Autodesk Inventor part; units mm, degrees
ref_plane "YZ Plane" through (0, 0, 0) normal (1, 0, 0) x (0, 1, 0)
ref_plane "XZ Plane" through (0, 0, 0) normal (0, 1, 0) x (-1, 0, 0)
ref_plane "XY Plane" through (0, 0, 0) normal (0, 0, 1) x (1, 0, 0)
sketch "Esquisse1" plane through (0, 0, 0) normal (0, 0, 1) x (1, 0, 0)
  line L0 (0, 0) -> (100, 0)
  line L1 (100, 0) -> (100, 80)
  line L2 (100, 80) -> (0, 80)
  line L3 (0, 80) -> (0, 0)
  dimension "d0" = 100
  dimension "d1" = 80
extrude "Extrusion1" add sketch "Esquisse1" against normal blind 5
sketch "Esquisse7" plane through (0, 0, 0) normal (0, 0, 1) x (1, 0, 0)
  line L0 (0, 0) -> (0, 45)
  line L1 (0, 0) -> (0, 80)
  line L2 (0, 45) -> (100, 45)
  line L3 (50, 45) -> (10, 45)
  line L4 (50, 45) -> (90, 45)
  line L5 (10, 45) -> (13, 45)
  line L6 (13, 45) -> (13, 50)
  line L7 (13, 50) -> (10, 50)
  line L8 (10, 50) -> (10, 45)
  line L9 (90, 45) -> (87, 45)
  line L10 (87, 45) -> (87, 50)
  line L11 (87, 50) -> (90, 50)
  line L12 (90, 50) -> (90, 45)
  line L13 (50, 45) -> (52.5, 45)
  line L14 (52.5, 45) -> (52.5, 50)
  line L15 (52.5, 50) -> (47.5, 50)
  line L16 (47.5, 50) -> (47.5, 45)
  line L17 (50, 45) -> (47.5, 45)
  line L18 (86.75, 44.75) -> (90.25, 44.75)
  line L19 (90.25, 44.75) -> (90.25, 50.25)
  line L20 (90.25, 50.25) -> (86.75, 50.25)
  line L21 (86.75, 50.25) -> (86.75, 44.75)
  line L22 (86.75, 44.75) -> (90.25, 50.25) construction
  line L23 (90.25, 44.75) -> (86.75, 50.25) construction
  line L24 (47.25, 44.75) -> (52.75, 44.75)
  line L25 (52.75, 44.75) -> (52.75, 50.25)
  line L26 (52.75, 50.25) -> (47.25, 50.25)
  line L27 (47.25, 50.25) -> (47.25, 44.75)
  line L28 (47.25, 44.75) -> (52.75, 50.25) construction
  line L29 (52.75, 44.75) -> (47.25, 50.25) construction
  line L30 (9.75, 44.75) -> (13.25, 44.75)
  line L31 (13.25, 44.75) -> (13.25, 50.25)
  line L32 (13.25, 50.25) -> (9.75, 50.25)
  line L33 (9.75, 50.25) -> (9.75, 44.75)
  line L34 (9.75, 44.75) -> (13.25, 50.25) construction
  line L35 (13.25, 44.75) -> (9.75, 50.25) construction
  point P0 (87, 45)
  point P1 (13, 45)
  point P2 (52.5, 45)
  point P3 (88.5, 47.5)
  point P4 (50, 47.5)
  point P5 (11.5, 47.5)
  point P6 (90.25, 45)
  point P7 (86.75, 45)
  point P8 (52.75, 45)
  point P9 (47.25, 45)
  point P10 (13.25, 45)
  point P11 (9.75, 45)
  point P12 (87, 45.05)
  point P13 (90, 45.05)
  dimension "d42" = 45
  dimension "d43" = 100
  dimension "d44" = 40
  dimension "d45" = 40
  dimension "d46" = 3
  dimension "d47" = 5
  dimension "d48" = 3
  dimension "d49" = 5
  dimension "d53" = 2.5
  dimension "d54" = 5
  dimension "d55" = 5
  dimension "d56" = 3.5
  dimension "d57" = 5.5
  dimension "d58" = 5.5
  dimension "d59" = 3.5
  dimension "d60" = 5.5
  dimension "d61" = 5.5
extrude "Extrusion2" cut sketch "Esquisse7" against normal through all
sketch "Esquisse8" plane through (0, 0, 0) normal (0, 0, 1) x (1, 0, 0)
  line L0 (0, 0) -> (0, 40)
  line L1 (0, 0) -> (0, 80)
  line L2 (0, 40) -> (50, 40)
  line L3 (100, 80) -> (100, 0)
  line L4 (-5, -5) -> (105, -5)
  line L5 (105, -5) -> (105, 85)
  line L6 (105, 85) -> (-5, 85)
  line L7 (-5, 85) -> (-5, -5)
  line L8 (-5, -5) -> (105, 85) construction
  line L9 (105, -5) -> (-5, 85) construction
  line L10 (100, 80) -> (0, 80)
  line L11 (0, 80) -> (0, 0)
  line L12 (0, 0) -> (100, 0)
  line L13 (100, 0) -> (100, 80)
  dimension "d62" = 40
  dimension "d63" = 50
  dimension "d64" = 110
  dimension "d65" = 90
extrude "Extrusion3" add sketch "Esquisse8" against normal blind 5
sketch "Esquisse9" plane through (0, 0, 0) normal (0, 0, 1) x (1, 0, 0)
  line L0 (0, 0) -> (-0.05, 0)
  line L1 (-0.05, 0) -> (-0.05, -0.95)
  line L2 (-0.05, -0.95) -> (20.05, -0.95)
  line L3 (20.05, -0.95) -> (20.05, -4.05)
  line L4 (20.05, -4.05) -> (-0.05, -4.05)
  line L5 (-0.05, -4.05) -> (-0.05, -0.95)
  line L6 (-5, -5) -> (105, -5)
  line L7 (105, -5) -> (50, -5)
  line L8 (50, -5) -> (50, 40.0521)
  line L9 (-5, -5) -> (-5, 85)
  line L10 (-5, 85) -> (-5, 40)
  line L11 (-5, 40) -> (20.05, 40)
  line L12 (100.05, -0.95) -> (79.95, -0.95)
  line L13 (79.95, -0.95) -> (79.95, -4.05)
  line L14 (79.95, -4.05) -> (100.05, -4.05)
  line L15 (100.05, -4.05) -> (100.05, -0.95)
  line L16 (-0.05, 80.95) -> (20.05, 80.95)
  line L17 (20.05, 80.95) -> (20.05, 84.05)
  line L18 (20.05, 84.05) -> (-0.05, 84.05)
  line L19 (-0.05, 84.05) -> (-0.05, 80.95)
  line L20 (100.05, 80.95) -> (79.95, 80.95)
  line L21 (79.95, 84.05) -> (100.05, 84.05)
  line L22 (79.95, 80.95) -> (79.95, 84.05)
  line L23 (100.05, 84.05) -> (100.05, 80.95)
  dimension "d68" = 0.05
  dimension "d69" = 0.95
  dimension "d70" = 20.1
  dimension "d71" = 3.1
  dimension "d72" = 55
  dimension "d73" = 45
extrude "Extrusion4" cut sketch "Esquisse9" against normal blind 5
sketch "Esquisse10" plane through (-5, 85, 0) normal (0, 1, 0) x (1, 0, 0)
  line L0 (110, 0) -> (0, 0)
  line L1 (110, 0) -> (110, 5)
  line L2 (0, 5) -> (110, 5)
  line L3 (0, 0) -> (0, 5)
  point P0 (5, 0)
extrude "Extrusion5" add sketch "Esquisse10" along normal blind 2
sketch "Esquisse11" plane through (-5, -5, 0) normal (0, -1, 0) x (1, 0, 0)
  line L0 (0, 0) -> (110, 0)
  line L1 (0, 0) -> (0, -5)
  line L2 (110, -5) -> (0, -5)
  line L3 (110, 0) -> (110, -5)
  point P0 (5, 0)
extrude "Extrusion6" add sketch "Esquisse11" along normal blind 2
properties part number "chassis arriere"
Design review of the part built by this model. Coordinates are the model's own, in mm. A direction names the side the tool comes from. Coordinates: 2 decimals unless noted, no trailing zeros. Loops run counter-clockwise (first coordinate to the right, second up) from the corner with the lowest first, then second, coordinate; pieces in that order, holes last. Notation, with made-up numbers: (32.25, -34) -> (85.25, -34) arc R11 cw to (85.25, -28) -> close; hole circle Ø11 at (74, -29). An arc over 180 degrees is marked (long way). Answer as a JSON object with one key per item and string values.
Q1. Tool access review of faces 3 (the flat face through (105, 41, -2)), 4 (the flat face through (47.25, 48, -2)): name each direction out of +Z, -Z, +X, -X, +Y, -Y from which nothing blocks a thin tool from reaching the whole face with its end or side.
Answer block:
{"face 3": "+Z, -Z, +X, +Y, -Y", "face 4": "+Z, -Z"}
Q2. The part is to be moulded in two halves that separate along Y. For faces 1 (the flat face through (51, 41, -5)), 2 (the flat face through (88, 44.75, -2)), say which applies: +Y half, -Y half, draft (parallel to the pull), parting line (faces both ways), or undercut.
Answer block:
{"face 1": "draft", "face 2": "undercut"}
Q3. Take a section at A-A on x = 7. Give the boundary of the cut face in (y, z), plus the area to 3 significant figures.
Answer block:
{"outline": "(-7, -5) -> (-4.05, -5) -> (-4.05, 0) -> (-7, 0) -> close; (-0.95, -5) -> (80.95, -5) -> (80.95, 0) -> (-0.95, 0) -> close; (84.05, -5) -> (87, -5) -> (87, 0) -> (84.05, 0) -> close", "area": "439 mm^2"}
Q4. Take a section at B-B on z = -3.4. Give the number of separate pieces and of enclosed holes in the cut face, plus the area to 3 significant figures.
Answer block:
{"separate pieces": "1", "enclosed holes": "7", "area": "10,000 mm^2"}
Q5. Take a section at C-C on x = 89. Give the boundary of the cut face in (y, z).
Answer block:
{"outline": "(-7, -5) -> (-4.05, -5) -> (-4.05, 0) -> (-7, 0) -> close; (-0.95, -5) -> (44.75, -5) -> (44.75, 0) -> (-0.95, 0) -> close; (50.25, -5) -> (80.95, -5) -> (80.95, 0) -> (50.25, 0) -> close; (84.05, -5) -> (87, -5) -> (87, 0) -> (84.05, 0) -> close"}
Q6. To check wall thickness, follow L1, parallel to Y at x = 90, z = -1.8; L2, parallel to Y at x = 7, z = -3.1; L3, parallel to X at y = 83, z = -1.8. State the ranges of each line that lie inside material, in increasing order.
Answer block:
{"L1": "y = -7 to -4.05, -0.95 to 44.75, 50.25 to 80.95, 84.05 to 87", "L2": "y = -7 to -4.05, -0.95 to 80.95, 84.05 to 87", "L3": "x = -5 to -0.05, 20.05 to 79.95, 100.05 to 105"}
